Check sheet for the modelled part. Datum: model origin and axes. Units: mm. A direction names the side the tool comes from. Round coordinates to 2 decimals unless told otherwise and drop trailing zeros. Loops run counter-clockwise (first coordinate to the right, second up) from the corner with the lowest first, then second, coordinate; pieces in that order, holes last. Notation, with made-up numbers: (21, 61.25) - (44, 61.25) arc R20 cw to (44, 80.25) - close; hole circle Ø9 at (25, 17). An arc over 180 degrees is marked (long way). Answer in a Markdown table with one row per item. Add a question column.
(1) Thickness scan on line 1 along Z through (x, y) = (-0.5, -3.75); line 2 along X through (y, z) = (-1.5, -1); line 3 along X through (y, z) = (-1.5, 0.25). Record the ranges inside material, lowest first.
(2) Mould release check, pull along Z, two halves, no side actions. Record for faces 1 (the cylindrical face through (-3.08, -4.96, 8.86)), 2 (the cylindrical face through (1.625, -6.472, -9.444)), 3 (the flat face through (-1, 0, -1)): +Z half, -Z half, draft (parallel to the pull), parting line (faces both ways), or undercut.
(3) Access from +Z, -Z, +X, -X, +Y, -Y to the whole of each face (thin tool, end or side, straight path). Record for faces 4 (the cylindrical face through (-0.378, -6.472, 2.054)), 5 (the flat face through (-1, -8, -1)).
(4) Cross-section at D-D on z = -3.25. Enter the section's corners in (x, y), then the cut area to 3 significant figures.
(5) Gauge pin test, flat ends, axial feed: pin 1 (1.5 mm diameter, centred on x = 1.5, z = 5, fed in from -Y); pin 2 (2 mm diameter, centred on x = 1, y = -4.5, fed in from -Z). Record the tip position at first contact, or that the pin passes through.
(6) Cross-section at C-C on y = -6.5. Enter the section's corners in (x, z), then the cut area to 3 significant figures.
(7) Cross-section at A-A on x = 5.5. Enter the section's corners in (y, z).
(8) Cross-section at B-B on z = 6. Enter the section's corners in (x, y), then the cut area to 3 significant figures.
from build123d import *

# Parameters (mm, degrees)
SKETCH2_R           = 9.9
BOSS_EXTRUDE1_DEPTH = 8
SKETCH2_3_R         = 12.75
BOSS_EXTRUDE2_DEPTH = 2
SKETCH2_4_R         = 1.65
CUT_EXTRUDE1_DEPTH  = 9
CUT_EXTRUDE2_START  = -8
SKETCH2_5_R         = 3
CUT_EXTRUDE2_DEPTH  = 3.1


with BuildPart() as part:
    # Sketch2 → Boss-Extrude1 (new body)
    with BuildSketch(Plane(origin=(0, 0, 0), x_dir=(1, 0, 0), z_dir=(0, 1, 0))):
        with Locations((-0.930712346, 0.804578045)):
            Circle(SKETCH2_R)
    extrude(amount=-BOSS_EXTRUDE1_DEPTH)

    # Sketch2<3> → Boss-Extrude2 (add)
    with BuildSketch(Plane(origin=(0, 0, 0), x_dir=(1, 0, 0), z_dir=(0, 1, 0))):
        with Locations((-0.930712346, 0.804578045)):
            Circle(SKETCH2_3_R)
    extrude(amount=-BOSS_EXTRUDE2_DEPTH)

    # Sketch2<4> → Cut-Extrude1 (cut, through all)
    with BuildSketch(Plane(origin=(0, 0, 0), x_dir=(1, 0, 0), z_dir=(0, 1, 0))):
        with Locations((0.012181629, 6.914065552)):
            Circle(SKETCH2_4_R)
        with Locations((0.012181629, -5.027976136)):
            Circle(SKETCH2_4_R)
        with Locations((-6.930712346, 0.804578045)):
            Circle(SKETCH2_4_R)
        with Locations((5.069287654, 0.804578045)):
            Circle(SKETCH2_4_R)
    extrude(amount=-CUT_EXTRUDE1_DEPTH, mode=Mode.SUBTRACT)

    # Sketch2<5> → Cut-Extrude2 (cut)
    with BuildSketch(Plane(origin=(0, 0, 0), x_dir=(1, 0, 0), z_dir=(0, 1, 0)).offset(CUT_EXTRUDE2_START)):
        with Locations((0.012181629, 6.914065552)):
            Circle(SKETCH2_5_R)
        with Locations((0.012181629, -5.027976136)):
            Circle(SKETCH2_5_R)
    extrude(amount=CUT_EXTRUDE2_DEPTH, mode=Mode.SUBTRACT)


solid = part.part
Answers:
| question | item | result |
|---|---|---|
| 1 | line 1 | z = -10.7 to -8.48, -5.35 to 3.46, 6.6 to 9.09 |
| 1 | line 2 | x = -13.68 to -8.57, -5.29 to 3.43, 6.71 to 11.82 |
| 1 | line 3 | x = -13.64 to -8.2, -5.66 to 3.8, 6.34 to 11.78 |
| 2 | face 1 | parting line |
| 2 | face 2 | undercut |
| 2 | face 3 | draft |
| 3 | face 4 | -Y |
| 3 | face 5 | +Z, -Z, +X, -X, -Y |
| 4 | outline | (-13.44, -2) - (-10.52, -2) - (-10.52, -8) - (8.66, -8) - (8.66, -2) - (11.58, -2) - (11.58, 0) - (-13.44, 0) - close |
| 4 | area | 165 mm^2 |
| 5 | pin 1 | stops at y = -4.9 |
| 5 | pin 2 | stops at z = -10.66 |
| 6 | outline | circle Ø19.8 at (-0.93, -0.8); hole circle Ø3.3 at (-6.93, -0.8); hole circle Ø6 at (0.01, -6.91); hole circle Ø6 at (0.01, 5.03); hole circle Ø3.3 at (5.07, -0.8) |
| 6 | area | 234 mm^2 |
| 7 | outline | (-8, -8.33) - (-2, -8.33) - (-2, -11.81) - (0, -11.81) - (0, -2.4) - (-8, -2.4) - close; (-8, 0.79) - (0, 0.79) - (0, 10.2) - (-2, 10.2) - (-2, 6.72) - (-8, 6.72) - close |
| 8 | outline | (-11.71, -2) - (-8.12, -2) - (-8.12, -8) - (-2.83, -8) - (-2.83, -4.9) - (-1.32, -4.9) - (-1.32, 0) - (-11.71, 0) - close; (1.35, -4.9) - (2.85, -4.9) - (2.85, -8) - (6.26, -8) - (6.26, -2) - (9.85, -2) - (9.85, 0) - (1.35, 0) - close |
| 8 | area | 98.8 mm^2 |
